Autodesk Inventor part; units mm, degrees
ref_plane "Work Plane5" through (0, 0, 101.6) normal (0, 0, 1) x (1, 0, 0)
ref_plane "Work Plane6" through (0, 0, 15.113) normal (0, 0, -1) x (-1, 0, 0)
ref_plane "Work Plane10" through (0, 0, 29.464) normal (0, 0, -1) x (-1, 0, 0)
sketch "Sketch1" plane through (0, 0, 0) normal (0, 0, 1) x (1, 0, 0)
  circle A0 centre (0, 0) radius 12.7
  circle A1 centre (0, 0) radius 6.35
  line L0 (-1.5875, 14.2875) -> (1.5875, 14.2875)
  line L1 (1.5875, 14.2875) -> (1.5875, 11.1125)
  line L2 (1.5875, 11.1125) -> (-1.5875, 11.1125)
  line L3 (-1.5875, 11.1125) -> (-1.5875, 14.2875)
  dimension "d0" = 25.4
  dimension "d4" = 12.7
  dimension "d50" = 3.175
  dimension "d51" = 3.175
  dimension "d52" = 1.5875
  dimension "d53" = 14.2875
extrude "Extrusion4" add sketch "Sketch1" along normal blind 104.775 contours A0 L3 L2 L1 | L1 L2 L3 A0
ref_plane "Work Plane5" through (0, 0, 101.6) normal (0, 0, 1) x (1, 0, 0)
sketch "Sketch6" plane through (0, 0, 101.6) normal (0, 0, 1) x (1, 0, 0)
  circle A0 centre (0, 0) radius 12.192
  circle A1 centre (0, 0) radius 12.7
  dimension "d24" = 24.384
extrude "Extrusion8" cut sketch "Sketch6" along normal blind 1.143
ref_plane "Work Plane6" through (0, 0, 15.113) normal (0, 0, -1) x (-1, 0, 0)
ref_plane "Work Plane9" through (0, 0, 43.3324) normal (0, 0, -1) x (-1, 0, 0)
ref_plane "Work Plane10" through (0, 0, 29.464) normal (0, 0, -1) x (-1, 0, 0)
extrude "Extrusion16" cut sketch "Sketch1" along normal through all contours L1 L2 L3 A0 | A0 L3 L0 L1 picked at (0.1768, 11.638)
sketch "Sketch14" plane through (0, 0, 104.775) normal (0, 0, 1) x (1, 0, 0)
  circle A0 centre (0, 0) radius 6.35
  circle A1 centre (0, 0) radius 7.9375
  dimension "d56" = 15.875
extrude "Extrusion17" cut sketch "Sketch14" against normal blind 7.9375
sketch "Sketch15" plane through (0, 0, 0) normal (0, 0, -1) x (-1, 0, 0)
  circle A0 centre (0, 0) radius 6.35
  circle A1 centre (0, 0) radius 7.9375
  dimension "d59" = 15.875
extrude "Extrusion18" cut sketch "Sketch15" against normal blind 7.9375
ref_plane "Work Plane13" through (0, 0, 6.35) normal (0, 0, -1) x (-1, 0, 0)
sketch "Sketch16" plane through (0, 0, 6.35) normal (0, 0, -1) x (-1, 0, 0)
  arc A0 (-1.5875, 12.6004) -> (1.5875, 12.6004) centre (0, 0) ccw
  line L0 (-1.5875, 12.6004) -> (-1.5875, 11.1125)
  line L1 (-1.5875, 11.1125) -> (1.5875, 11.1125)
  line L2 (1.5875, 11.1125) -> (1.5875, 12.6004)
  circle A1 centre (0, 0) radius 15.875
  circle A2 centre (0, 0) radius 14.2875
  dimension "d63" = 31.75
  dimension "d68" = 28.575
extrude "Extrusion19" add sketch "Sketch16" against normal blind 3.175 contours A1 | A2
sketch "Sketch17" plane through (0, 0, 0) normal (0, 0, -1) x (-1, 0, 0)
  line L0 (-1.5875, 11.1125) -> (-1.5875, 12.6004)
  arc A0 (-1.5875, 12.6004) -> (1.5875, 12.6004) centre (0, 0) ccw
  line L1 (1.5875, 12.6004) -> (1.5875, 11.1125)
  line L2 (1.5875, 11.1125) -> (-1.5875, 11.1125)
  arc A1 (1.5875, 12.6004) -> (-1.5875, 12.6004) centre (0, 0) ccw
extrude "Extrusion20" add sketch "Sketch17" against normal blind 6.35 contours L0 A1 L1 L2
extrude "Extrusion21" add sketch "Sketch16" against normal blind 6.35 contours A2
equation "\"d51\" = d50"
properties part number "turn shaft 2"
Check sheet for the modelled part. Datum: model origin and axes. Units: mm. A direction names the side the tool comes from. Give positions to 0.01 mm unless a question says otherwise; leave off trailing zeros. Write each loop counter-clockwise with the first axis right and the second up, starting at its lowest first coordinate (ties: lowest second). Pieces come first, ordered by that corner, then holes. Notation, with made-up numbers: (-8, 87.25) -> (27, 87.25) arc R22 cw to (27, 124.25) -> close; hole circle Ø9 at (1, 85). An arc over 180 degrees is marked (long way). Use one line per item in the form item = value. Start each with the question number.
1. Mould release check, pull along Y, two halves, no side actions. Record for faces 1 (the flat face through (-8.3, 0.2, 0)), 2 (the flat face through (0, 7, 7.938)), 3 (the flat face through (0, 7, 96.838)), 4 (the cylindrical face through (0.54, -12.69, 103.74)): pulls with the +Y half, pulls with the -Y half, needs draft (parallel to the pull), parting line crosses it, or undercut.
2. Go/stop test with flat-tipped pins: P1, Ø14.5, axis at x = 0, y = 0, coming from the +Z side; P2, Ø12.5, axis at x = 3, y = 3.5, coming from the +Z side (3 decimals); P3, Ø10, axis at y = 11.5, z = 42, coming from the +X side; P4, Ø2.5, axis at x = 0.5, z = 78.5, coming from the +Y side. Record where each tip stops, or that it passes through.
3. Section check B-B (z = 41). Record the cut outline in (x, y).
4. Thickness scan on line 1 along Y through (x, z) = (0, 102.5); line 2 along Z through (x, y) = (13, 4.5); line 3 along Y through (x, z) = (0, 101). Record the ranges inside material, lowest first. Write a range as from..to.
5. Access from +Z, -Z, +X, -X, +Y, -Y to the whole of each face (thin tool, end or side, straight path). Record for faces 5 (the flat face through (-12.3, -1.9, 101.6)), 6 (the cylindrical face through (3.441, -15.497, 7.915)), 7 (the flat face through (0, 11.112, 58)), 8 (the flat face through (1, 12, 12.7)), 9 (the flat face through (7, 11, 6.35)).
Conclusion:
q1.face_1 = needs draft
q1.face_2 = undercut
q1.face_3 = undercut
q1.face_4 = parting line crosses it
q2.P1 = 96.84
q2.P2 = 104.775
q2.P3 = 10.91
q2.P4 = 12.6
q3.outline = (-1.59, 11.11) -> (-1.59, 12.6) arc R12.7 ccw (long way) to (1.59, 12.6) -> (1.59, 11.11) -> close; hole circle Ø12.7 at (0, 0)
q4.line_1 = -12.19..-7.94, 7.94..11.11
q4.line_2 = 6.35..12.7
q4.line_3 = -12.7..-7.94, 7.94..11.11
q5.face_5 = none
q5.face_6 = +Z, -Z
q5.face_7 = +Z, +Y
q5.face_8 = +Z
q5.face_9 = -Z
